Study the drawing (mm; zero at the part's minimum x, y, z) and answer. A direction names the side the tool comes from. Coordinates: 2 decimals unless noted, no trailing zeros. Loops run counter-clockwise (first coordinate to the right, second up) from the corner with the lowest first, then second, coordinate; pieces in that order, holes last. Notation, with made-up numbers: (-31.75, -12) - (-8.75, -12) arc R17 cw to (-8.75, -3) - close; hole circle Ø3 at (23, -21.75). An arc over 180 degrees is marked (long way). Put each result on its own line as item: value.
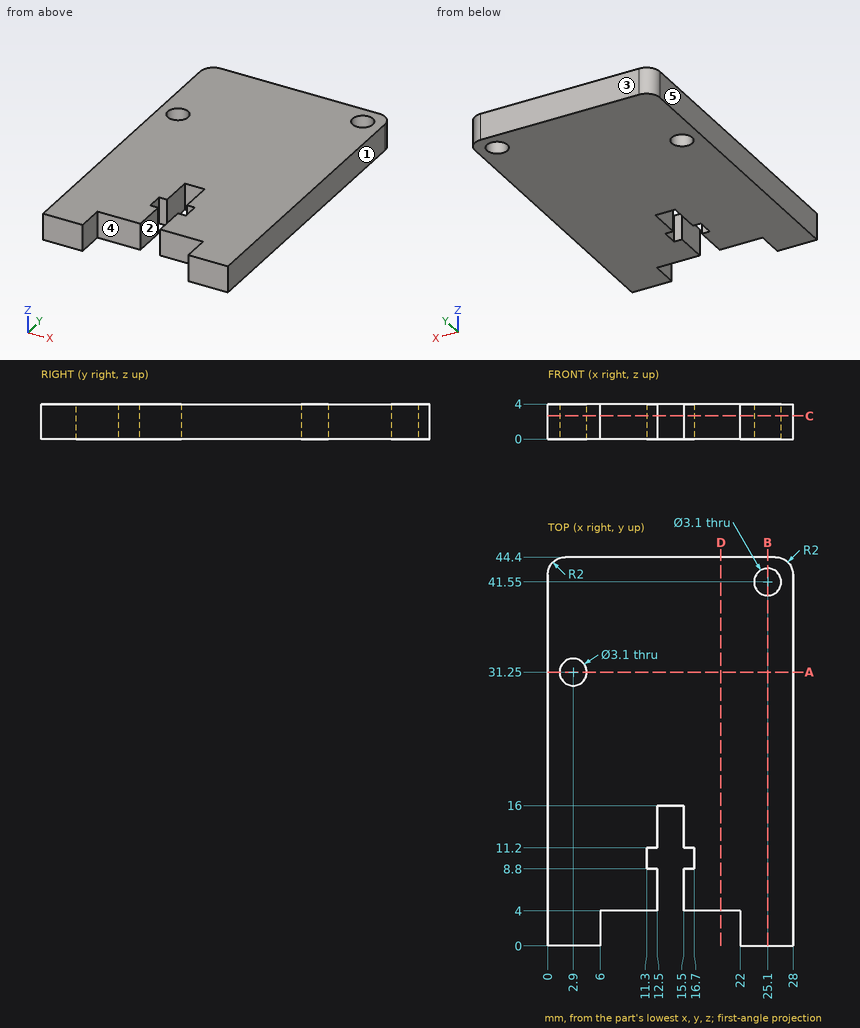
1) The part is cut by section B-B (x = 25.1). Give the vertices of the cut face in (y, z), and give its area (3 significant figures).
Found:
outline: (0, 0) - (40, 0) - (40, 4) - (0, 4) - close; (43.1, 0) - (44.4, 0) - (44.4, 4) - (43.1, 4) - close
area: 165 mm^2
2) Straight lines are drawn through the part: L1, parallel to Y at x = 25.1, z = 2.95; L2, parallel to Y at x = 2.9, z = 1.2; L3, parallel to X at y = 15, z = 3.55. For each, find the intervals that lie inside material, in ascending order. Write a range as [from, to].
Found:
L1: y = [0, 40], [43.1, 44.4]
L2: y = [0, 29.7], [32.8, 44.4]
L3: x = [0, 12.5], [15.5, 28]
3) For the marked faces 1 and 2, determine the directions among +Z, -Z, +X, -X, +Y, -Y from which every point of the face is accessible in a straight line to the end or side of a thin tool.
Found:
face 1: +Z, -Z, +X, +Y, -Y
face 2: +Z, -Z, -Y
4) The part is cut by section C-C (z = 2.65). Give the vertices of the cut face in (x, y), and give its area (3 significant figures).
Found:
outline: (0, 0) - (6, 0) - (6, 4) - (12.5, 4) - (12.5, 8.8) - (11.3, 8.8) - (11.3, 11.2) - (12.5, 11.2) - (12.5, 16) - (15.5, 16) - (15.5, 11.2) - (16.7, 11.2) - (16.7, 8.8) - (15.5, 8.8) - (15.5, 4) - (22, 4) - (22, 0) - (28, 0) - (28, 42.4) arc R2 ccw to (26, 44.4) - (2, 44.4) arc R2 ccw to (0, 42.4) - close; hole circle Ø3.1 at (2.9, 31.25); hole circle Ø3.1 at (25.1, 41.55)
area: 1,120 mm^2
5) The part is cut by section A-A (y = 31.25). Give the vertices of the cut face in (x, z).
Found:
outline: (0, 0) - (1.35, 0) - (1.35, 4) - (0, 4) - close; (4.45, 0) - (28, 0) - (28, 4) - (4.45, 4) - close
6) This flat-tipped pin is pushed along its axis until it touches: pin 1 (1.2 mm diameter, centred on x = 9, z = 1.5, fed in from -Y). Where does it stop, or does it pass through?
Found:
pin 1: stops at y = 4
7) For a pull along X with two mould halves and no side action, classify the marked faces 3, 4 and 5 as pulls with the +X half, pulls with the -X half, needs draft (parallel to the pull), parting line crosses it, or undercut.
Found:
face 3: needs draft
face 4: undercut
face 5: pulls with the -X half
8) The part is cut by section D-D (x = 19.75). Give the vertices of the cut face in (y, z), and give its area (3 significant figures).
Found:
outline: (4, 0) - (44.4, 0) - (44.4, 4) - (4, 4) - close
area: 162 mm^2
